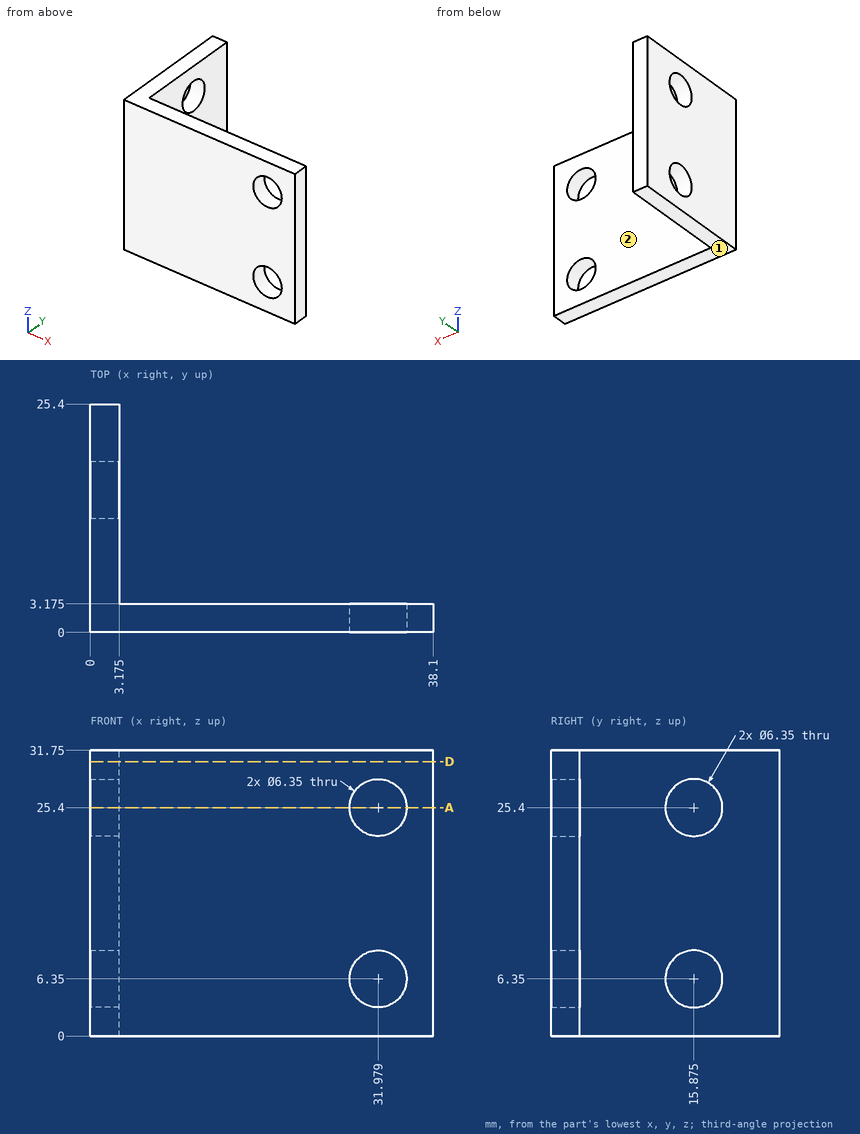
For this review, use the dimensioned drawing (mm, ordinates from the lowest corner) and the shaded views. A direction names the side the tool comes from. Coordinates: 2 decimals unless noted, no trailing zeros. Loops run counter-clockwise (first coordinate to the right, second up) from the corner with the lowest first, then second, coordinate; pieces in that order, holes last. Notation, with made-up numbers: (42, 73) -> (74, 73) arc R18 cw to (74, 83) -> close; hole circle Ø11 at (10.25, -4). An arc over 180 degrees is marked (long way). Return JSON: item names as keys, results as strings. Group by question number.
(1) For pin 1 Ø4 at (y, z) = (22.5, 3.5) entering from +X (3 decimals); pin 2 Ø5.5 at (y, z) = (15.875, 25.4) entering from -X; pin 3 Ø10 at (x, z) = (31.98, 25.4) entering from +Y (3 decimals), all flat-tipped, find the tip position at first contact; note any pin that passes through.
(2) Consider section A-A, the plane z = 25.4. Count the separate pieces of the cut face and the enclosed holes in it, plus the area to 3 significant figures.
(3) To check wall thickness, follow L1, parallel to Z at x = 2.5, y = 17; L2, parallel to X at y = 1.2, z = 25.4; L3, parallel to Y at x = 1.7, z = 6.35. State the ranges of each line that lie inside material, in increasing order.
(4) Consider section D-D, the plane z = 30.5. Give the boundary of the cut face in (x, y) (1 decimal).
(5) Tool access review of the marked faces 1 and 2: name each direction out of +Z, -Z, +X, -X, +Y, -Y from which nothing blocks a thin tool from reaching the whole face with its end or side.
Results below:
{
 "1": {"pin 1": "stops at x = 3.175", "pin 2": "passes through", "pin 3": "stops at y = 3.175"},
 "2": {"separate pieces": "3", "enclosed holes": "0", "area": "151 mm2"},
 "3": {"L1": "z = 0 to 3.38, 9.32 to 22.43, 28.37 to 31.75", "L2": "x = 0 to 28.8, 35.15 to 38.1", "L3": "y = 0 to 12.7, 19.05 to 25.4"},
 "4": {"outline": "(0, 0) -> (38.1, 0) -> (38.1, 3.2) -> (3.2, 3.2) -> (3.2, 25.4) -> (0, 25.4) -> close"},
 "5": {"face 1": "-Z, +X, -X, +Y, -Y", "face 2": "+Z, -Z, +X, +Y"}
}
